Part model, mm, in its own coordinate system. Coordinates: 2 decimals unless noted, no trailing zeros. Order: outer loops, then holes, each group sorted by start corner. A loop starts at its lowest first (then second) coordinate and runs counter-clockwise, first axis right, second up.
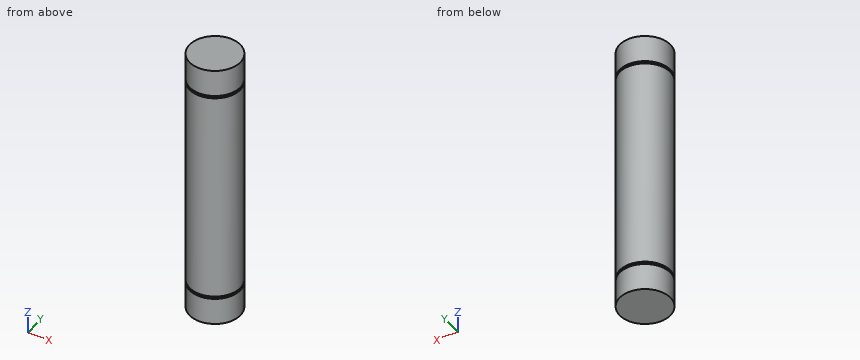
from build123d import *

# Parameters (mm, degrees)
SKETCH1_R           = 14.29004
BOSS_EXTRUDE1_DEPTH = 76.2
SKETCH2_W           = 1.4224
SKETCH2_H           = 0.84074


with BuildPart() as part:
    # Sketch1 → Boss-Extrude1 (new, symmetric)
    with BuildSketch(Plane.XY):
        Circle(SKETCH1_R)
    extrude(amount=BOSS_EXTRUDE1_DEPTH, both=True)

    # Sketch2 → Cut-Revolve1 (revolve, cut)
    with BuildSketch(Plane(origin=(0, 0, 0), x_dir=(0, 0, -1), z_dir=(1, 0, 0)), mode=Mode.PRIVATE) as cut_revolve1_sk:
        with Locations((-60.4012, 13.86967)):
            Rectangle(SKETCH2_W, SKETCH2_H)
    cut_revolve1 = revolve(cut_revolve1_sk.sketch.rotate(Axis((0, 0, 76.2), (0, 0, -1)), 90), axis=Axis((0, 0, 76.2), (0, 0, -1)), mode=Mode.SUBTRACT)

    # Mirror1: Cut-Revolve1 across plane
    add(cut_revolve1.mirror(Plane.XY), mode=Mode.SUBTRACT)


solid = part.part
Q1. Cut at C-C on z = -35.5. Write the cut outline in (x, y).
Results list:
outline: circle Ø28.58 at (0, 0)
Q2. Pin check, flat tips, straight feed: pin 1 Ø5 at (y, z) = (-6, 14.5) entering from +X; pin 2 Ø6 at (x, z) = (-3.5, -46) entering from -Y; pin 3 Ø1 at (y, z) = (-10, 2) entering from -X (3 decimals). Stop position of each tip, or through.
Results list:
pin 1: stops at x = 13.85
pin 2: stops at y = -14.28
pin 3: stops at x = -10.675
Q3. Cut at B-B on y = 3.5. Write the cut outline in (x, z).
Results list:
outline: (-13.85, -76.2) - (13.85, -76.2) - (13.85, -61.11) - (12.99, -61.11) - (12.99, -59.69) - (13.85, -59.69) - (13.85, 59.69) - (12.99, 59.69) - (12.99, 61.11) - (13.85, 61.11) - (13.85, 76.2) - (-13.85, 76.2) - (-13.85, 61.11) - (-12.99, 61.11) - (-12.99, 59.69) - (-13.85, 59.69) - (-13.85, -59.69) - (-12.99, -59.69) - (-12.99, -61.11) - (-13.85, -61.11) - close
Q4. Wall check: line 1 along Y through (x, z) = (-0.75, -49); line 2 along X through (y, z) = (4.75, -15.5); line 3 along X through (y, z) = (12.5, -61.5). Give the ranges that are in metal, low to high.
Results list:
line 1: y = -14.27 to 14.27
line 2: x = -13.48 to 13.48
line 3: x = -6.92 to 6.92
Q5. Cut at A-A on x = -6.5. Write the cut outline in (y, z).
Results list:
outline: (-12.73, -76.2) - (12.73, -76.2) - (12.73, -61.11) - (11.77, -61.11) - (11.77, -59.69) - (12.73, -59.69) - (12.73, 59.69) - (11.77, 59.69) - (11.77, 61.11) - (12.73, 61.11) - (12.73, 76.2) - (-12.73, 76.2) - (-12.73, 61.11) - (-11.77, 61.11) - (-11.77, 59.69) - (-12.73, 59.69) - (-12.73, -59.69) - (-11.77, -59.69) - (-11.77, -61.11) - (-12.73, -61.11) - close
